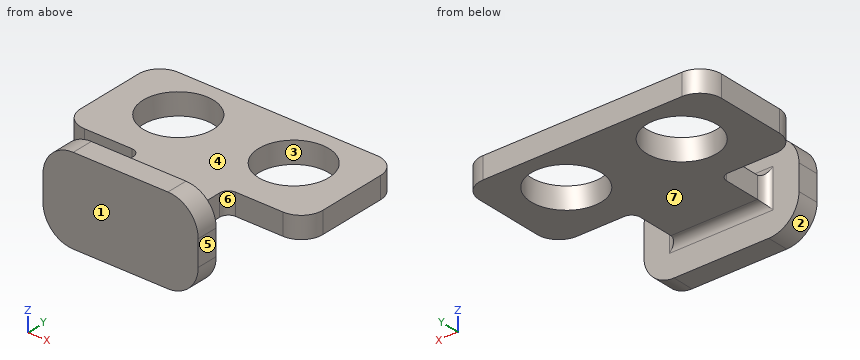
from build123d import *

# Parameters (mm, degrees)
SKETCH1_W           = 3
SKETCH1_H           = 23
SKETCH1_W_2         = 56
SKETCH1_H_2         = 3
BOSS_EXTRUDE1_DEPTH = 5
SKETCH7_W           = 20
SKETCH7_H           = 5
BOSS_EXTRUDE7_DEPTH = 12.5
SKETCH8_W           = 35.9
SKETCH8_H           = 19.9
BOSS_EXTRUDE8_DEPTH = 5
FILLET3_R           = 5
FILLET5_R           = 2
FILLET9_R           = 2
FILLET10_R          = 7


with BuildPart() as part:
    # Sketch1 → Boss-Extrude1 (new body)
    with BuildSketch(Plane.XY):
        with BuildLine():
            Line((50, 11.5), (46.45, 11.5))
            ThreePointArc((46.45, 11.5), (38.35, 3.4), (30.25, 11.5))
            Line((30.25, 11.5), (19.75, 11.5))
            ThreePointArc((19.75, 11.5), (11.65, 3.4), (3.55, 11.5))
            Line((3.55, 11.5), (0, 11.5))
            Line((0, 11.5), (0, 0))
            Line((0, 0), (50, 0))
            Line((50, 0), (50, 11.5))
        make_face()
        with BuildLine():
            ThreePointArc((30.25, 11.5), (38.35, 19.6), (46.45, 11.5))
            Line((46.45, 11.5), (50, 11.5))
            Line((50, 11.5), (50, 23))
            Line((50, 23), (0, 23))
            Line((0, 23), (0, 11.5))
            Line((0, 11.5), (3.55, 11.5))
            ThreePointArc((3.55, 11.5), (11.65, 19.6), (19.75, 11.5))
            Line((19.75, 11.5), (30.25, 11.5))
        make_face()
        with Locations((-1.5, 11.5)):
            Rectangle(SKETCH1_W, SKETCH1_H)
        with Locations((51.5, 11.5)):
            Rectangle(SKETCH1_W, SKETCH1_H)
        with Locations((25, -1.5)):
            Rectangle(SKETCH1_W_2, SKETCH1_H_2)
    extrude(amount=BOSS_EXTRUDE1_DEPTH)

    # Sketch7 → Boss-Extrude7 (add)
    with BuildSketch(Plane.XZ.offset(3)):
        with Locations((25, 2.5)):
            Rectangle(SKETCH7_W, SKETCH7_H)
    extrude(amount=BOSS_EXTRUDE7_DEPTH)

    # Sketch8 → Boss-Extrude8 (add)
    with BuildSketch(Plane.XZ.offset(15.5)):
        with Locations((25, 2.5)):
            Rectangle(SKETCH8_W, SKETCH8_H)
    extrude(amount=BOSS_EXTRUDE8_DEPTH)

    # Fillet3
    fillet3_edges = [part.edges().sort_by_distance(p)[0] for p in [
        (53, 23, 2.5),
        (-3, 23, 2.5),
        (53, -3, 2.5),
        (-3, -3, 2.5),
    ]]
    fillet(fillet3_edges, radius=FILLET3_R)

    # Fillet5
    fillet5_edges = [part.edges().sort_by_distance(p)[0] for p in [
        (35, -3, 2.5),
        (15, -3, 2.5),
    ]]
    fillet(fillet5_edges, radius=FILLET5_R)

    # Fillet9
    fillet9_edges = [part.edges().sort_by_distance(p)[0] for p in [
        (35, -15.5, 2.5),
        (25, -15.5, 5),
        (15, -15.5, 2.5),
        (25, -15.5, 0),
    ]]
    fillet(fillet9_edges, radius=FILLET9_R)

    # Fillet10
    fillet10_edges = [part.edges().sort_by_distance(p)[0] for p in [
        (42.95, -18, -7.45),
        (42.95, -18, 12.45),
        (7.05, -18, 12.45),
        (7.05, -18, -7.45),
    ]]
    fillet(fillet10_edges, radius=FILLET10_R)


solid = part.part
Design review of the part built by this model. Coordinates are the model's own, in mm. Face numbers are marked on the shaded views. A direction names the side the tool comes from. Round coordinates to 2 decimals unless told otherwise and drop trailing zeros. Loops run counter-clockwise (first coordinate to the right, second up) from the corner with the lowest first, then second, coordinate; pieces in that order, holes last. Notation, with made-up numbers: (45.5, 48.25) - (94.5, 48.25) arc R27 cw to (94.5, 68.25) - close; hole circle Ø2 at (42, 71). An arc over 180 degrees is marked (long way). One line per item, written item: value. Start each with the question number.
1) Consider section C-C on x = 34. Give the boundary of the cut face in (y, z).
2) Draft analysis for pull direction Y (two halves, no side actions). For the marked faces 1, 2 and 3, state which applies: +Y half, -Y half, draft (parallel to the pull), parting line (faces both ways), or undercut.
3) To check wall thickness, follow L1, parallel to Y at x = 38.35, z = 2.45; L2, parallel to X at y = 5, z = 3.25; L3, parallel to X at y = 4.5, z = 0.75. State the ranges of each line that lie inside material, in increasing order. Write a range as from..to.
4) Consider section D-D on y = 4. Give the boundary of the cut face in (x, z).
5) Consider section A-A on y = 11.5. Give the boundary of the cut face in (x, z).
6) Consider section B-B on x = 25.5. Give the boundary of the cut face in (y, z).
7) For the marked faces 4, 5, 6 and 7, list the 3-axis set-ups (+Z, -Z, +X, -X, +Y, -Y) from which the entire face can be reached by the end or side of a thin tool; tool diameter is ignored.
8) Insertion check: pin 1 Ø4 at (y, z) = (-17, 3.5) entering from -X; pin 2 Ø18 at (x, y) = (30.5, 1) entering from +Z; pin 3 Ø1 at (x, y) = (35, 16.5) entering from -Z; pin 4 Ø2.5 at (y, z) = (-17.5, 2.5) entering from +X. Each pin has a flat end and moves straight along its axis. Give the tip position at first contact, or say it passes through.
Reported:
1. outline: (-20.5, -7.45) - (-15.5, -7.45) - (-15.5, -2) arc R2 cw to (-13.5, 0) - (4.67, 0) - (4.67, 5) - (-13.5, 5) arc R2 cw to (-15.5, 7) - (-15.5, 12.45) - (-20.5, 12.45) - close; (18.33, 0) - (23, 0) - (23, 5) - (18.33, 5) - close
2. face 1: -Y half
2. face 2: draft
2. face 3: undercut
3. L1: y = -20.5..-15.5, -3..3.4, 19.6..23
3. L2: x = -3..6.82, 16.48..33.52, 43.18..53
3. L3: x = -3..7.57, 15.73..34.27, 42.43..53
4. outline: (-3, 0) - (8.59, 0) - (8.59, 5) - (-3, 5) - close; (14.71, 0) - (35.29, 0) - (35.29, 5) - (14.71, 5) - close; (41.41, 0) - (53, 0) - (53, 5) - (41.41, 5) - close
5. outline: (-3, 0) - (3.55, 0) - (3.55, 5) - (-3, 5) - close; (19.75, 0) - (30.25, 0) - (30.25, 5) - (19.75, 5) - close; (46.45, 0) - (53, 0) - (53, 5) - (46.45, 5) - close
6. outline: (-20.5, -7.45) - (-15.5, -7.45) - (-15.5, -2) arc R2 cw to (-13.5, 0) - (23, 0) - (23, 5) - (-13.5, 5) arc R2 cw to (-15.5, 7) - (-15.5, 12.45) - (-20.5, 12.45) - close
7. face 4: +Z, +X, -X, +Y
7. face 5: +Z, -Z, +X, -Y
7. face 6: +Z, -Z, +X
7. face 7: -Z, +X, -X, +Y
8. pin 1: stops at x = 7.05
8. pin 2: stops at z = 5
8. pin 3: passes through
8. pin 4: stops at x = 42.95
